```python
from build123d import *

# Parameters (mm, degrees)
BOSS_EXTRUDE1_DEPTH = 20
SKETCH2_W           = 2.639320226
SKETCH2_H           = 10
CUT_EXTRUDE1_DEPTH  = 20


with BuildPart() as part:
    # Sketch1 → Boss-Extrude1 (new body)
    with BuildSketch(Plane(origin=(0, 0, 0), x_dir=(0, 1, 0), z_dir=(0, 0, 1))):
        with BuildLine():
            Line((0, 0), (5, 0))
            Line((5, 0), (5, 10))
            Line((5, 10), (25, 10))
            Line((25, 10), (25, 0))
            Line((25, 0), (30, 0))
            ThreePointArc((30, 0), (15, 15), (0, 0))
        make_face()
    extrude(amount=BOSS_EXTRUDE1_DEPTH)

    # Sketch2 → Cut-Extrude1 (cut)
    with BuildSketch(Plane.XY.offset(20)):
        with Locations((-12.5, 15)):
            Rectangle(SKETCH2_W, SKETCH2_H)
    extrude(amount=-CUT_EXTRUDE1_DEPTH, mode=Mode.SUBTRACT)


solid = part.part
```
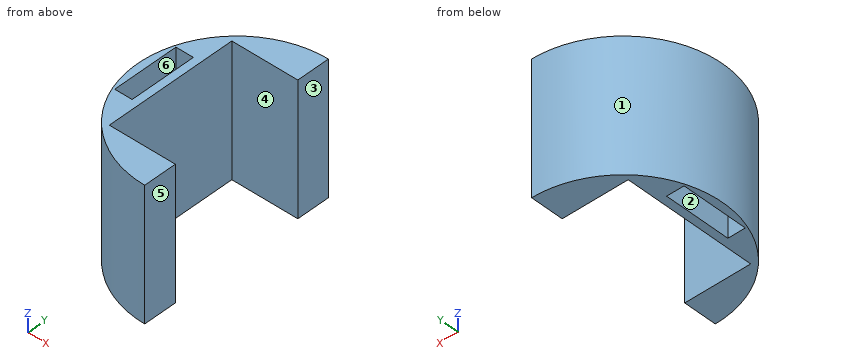
Can you work these out from the model? Positions are in its coordinate system, mm. Face numbers are marked on the shaded views. A direction names the side the tool comes from. Round coordinates to 2 decimals unless told otherwise and drop trailing zeros. Loops run counter-clockwise (first coordinate to the right, second up) from the corner with the lowest first, then second, coordinate; pieces in that order, holes last. Notation, with made-up numbers: (-28, 39) -> (3, 39) arc R28 cw to (3, 76) -> close; hole circle Ø8 at (24, 48.25). An arc over 180 degrees is marked (long way). Answer in a Markdown table with one row per item.
Item 1: Suppose I cut it at C-C, the plane z = 12.25. List the corners of the cut face in (x, y) for me.
Answer block:
| item | result |
|---|---|
| outline | (-10, 5) -> (-10, 25) -> (0, 25) -> (0, 30) arc R15 ccw to (0, 0) -> (0, 5) -> close; hole (-13.82, 10) -> (-11.18, 10) -> (-11.18, 20) -> (-13.82, 20) -> close |
Item 2: Will these pins go through, and if not, where does the flat tip stop? P1, Ø1, axis at y = 26, z = 13, coming from the -X side; P2, Ø4, axis at x = -7, z = 8, coming from the +Y side; P3, Ø8, axis at x = -5.5, z = 7.5, coming from the +Y side.
Answer block:
| item | result |
|---|---|
| P1 | x = -10.71 |
| P2 | y = 29.14 |
| P3 | y = 29.92 |
Item 3: If I drill on probe 1 along Y at (x, z) = (-7, 3.5); probe 2 along X at (y, z) = (14.5, 16); probe 3 along X at (y, z) = (18.25, 4.75), over which ranges is the centre line in solid material (lowest first)?
Answer block:
| item | result |
|---|---|
| probe 1 | 1.73 to 5, 25 to 28.27 |
| probe 2 | -14.99 to -13.82, -11.18 to -10 |
| probe 3 | -14.64 to -13.82, -11.18 to -10 |
Item 4: On a 3-axis mill with a long thin cutter (end or side, diameter ignored), from which of +Z, -Z, +X, -X, +Y, -Y can I reach the whole of each face in a straight line? I mean the marked faces 4, 5 and 6. Say none if no direction works.
Answer block:
| item | result |
|---|---|
| face 4 | +Z, -Z, +X |
| face 5 | +Z, -Z, +X, +Y, -Y |
| face 6 | +Z, -Z |
Item 5: Suppose I cut it at D-D, the plane y = 20.75. List the corners of the cut face in (x, z) for me.
Answer block:
| item | result |
|---|---|
| outline | (-13.85, 0) -> (-10, 0) -> (-10, 20) -> (-13.85, 20) -> close |
Item 6: Suppose I cut it at A-A, the plane y = 15. List the corners of the cut face in (x, z) for me.
Answer block:
| item | result |
|---|---|
| outline | (-15, 0) -> (-13.82, 0) -> (-13.82, 20) -> (-15, 20) -> close; (-11.18, 0) -> (-10, 0) -> (-10, 20) -> (-11.18, 20) -> close |
Item 7: Suppose I cut it at B-B, the plane x = -5.5. List the corners of the cut face in (y, z) for me, plus the area to 3 significant figures.
Answer block:
| item | result |
|---|---|
| outline | (1.04, 0) -> (5, 0) -> (5, 20) -> (1.04, 20) -> close; (25, 0) -> (28.96, 0) -> (28.96, 20) -> (25, 20) -> close |
| area | 158 mm² |
Item 8: We'd pull the mould along Y, two halves only. Please class the marked faces 1, 2 and 3: released by +Y, released by -Y, zero draft, split by the parting line, or undercut.
Answer block:
| item | result |
|---|---|
| face 1 | split by the parting line |
| face 2 | undercut |
| face 3 | zero draft |
